```python
from build123d import *

# Parameters (mm, degrees)
SKETCH1_W           = 14.1
SKETCH1_H           = 31.1
BOSS_EXTRUDE1_DEPTH = 1.5
SKETCH2_W           = 10
SKETCH2_H           = 5.6
BOSS_EXTRUDE2_DEPTH = 9
SKETCH3_W           = 0.5
SKETCH3_H           = 5.6
BOSS_EXTRUDE3_DEPTH = 2.3
SKETCH4_R           = 1.5
BOSS_EXTRUDE4_DEPTH = 1.7
CHAMFER1_SIZE       = 1
CHAMFER2_SIZE       = 0.5
FILLET1_R           = 1
FILLET2_R           = 1
SKETCH5_R           = 0.4
BOSS_EXTRUDE5_DEPTH = 1
SKETCH6_R           = 1.5
CUT_EXTRUDE1_DEPTH  = 11


with BuildPart() as part:
    # Sketch1 → Boss-Extrude1 (new body)
    with BuildSketch(Plane(origin=(0, 0, 0), x_dir=(1, 0, 0), z_dir=(0, 1, 0))):
        Rectangle(SKETCH1_W, SKETCH1_H)
    extrude(amount=BOSS_EXTRUDE1_DEPTH)

    # Sketch2 → Boss-Extrude2 (add)
    with BuildSketch(Plane(origin=(0, 1.5, 0), x_dir=(1, 0, 0), z_dir=(0, 1, 0))):
        with Locations((0, 11.95)):
            Rectangle(SKETCH2_W, SKETCH2_H)
    extrude(amount=BOSS_EXTRUDE2_DEPTH)

    # Sketch3 → Boss-Extrude3 (add)
    with BuildSketch(Plane(origin=(0, 10.5, 0), x_dir=(1, 0, 0), z_dir=(0, 1, 0))):
        with Locations((0, 11.95)):
            Rectangle(SKETCH3_W, SKETCH3_H)
    extrude(amount=BOSS_EXTRUDE3_DEPTH)

    # Sketch4 → Boss-Extrude4 (add)
    with BuildSketch(Plane(origin=(0, 10.5, 0), x_dir=(1, 0, 0), z_dir=(0, 1, 0))):
        with Locations(Location((-2.625, 11.95, 0), (0, 0, 270))):
            Circle(SKETCH4_R)
        with Locations(Location((2.625, 11.95, 0), (0, 0, 270))):
            Circle(SKETCH4_R)
    extrude(amount=BOSS_EXTRUDE4_DEPTH)

    # Chamfer1
    chamfer1_edges = [part.edges().sort_by_distance(p)[0] for p in [
        (5, 6, -9.15),
        (5, 6, -14.75),
        (-5, 6, -14.75),
        (-5, 6, -9.15),
    ]]
    chamfer(chamfer1_edges, length=CHAMFER1_SIZE)

    # Chamfer2
    chamfer2_edges = [part.edges().sort_by_distance(p)[0] for p in [
        (-2.125, 10.5, -14.75),
        (2.125, 10.5, -9.15),
        (-5, 10.5, -11.95),
        (2.125, 10.5, -14.75),
        (-2.125, 10.5, -9.15),
        (-4.5, 10.5, -9.65),
        (-4.5, 10.5, -14.25),
        (5, 10.5, -11.95),
        (4.5, 10.5, -14.25),
        (4.5, 10.5, -9.65),
    ]]
    chamfer(chamfer2_edges, length=CHAMFER2_SIZE)

    # Fillet1
    fillet1_edges = [part.edges().sort_by_distance(p)[0] for p in [
        (-2.625, 12.2, -13.45),
        (2.625, 12.2, -13.45),
    ]]
    fillet(fillet1_edges, radius=FILLET1_R)

    # Fillet2
    fillet2_edges = [part.edges().sort_by_distance(p)[0] for p in [
        (0, 12.8, -14.75),
        (0, 12.8, -9.15),
    ]]
    fillet(fillet2_edges, radius=FILLET2_R)

    # Sketch5 → Boss-Extrude5 (add)
    with BuildSketch(Plane(origin=(0, 1.5, 0), x_dir=(1, 0, 0), z_dir=(0, 1, 0))):
        with Locations(Location((-4.05, 1.85, 0), (0, 0, 270))):
            Circle(SKETCH5_R)
        with Locations(Location((-1.55, -0.45, 0), (0, 0, 270))):
            Circle(SKETCH5_R)
        with Locations(Location((-4.05, -2.75, 0), (0, 0, 270))):
            Circle(SKETCH5_R)
        with Locations(Location((-3.84, -14.05, 0), (0, 0, 270))):
            Circle(SKETCH5_R)
        with Locations(Location((-1.28, -14.05, 0), (0, 0, 270))):
            Circle(SKETCH5_R)
        with Locations(Location((1.28, -14.05, 0), (0, 0, 270))):
            Circle(SKETCH5_R)
        with Locations(Location((3.84, -14.05, 0), (0, 0, 270))):
            Circle(SKETCH5_R)
    extrude(amount=BOSS_EXTRUDE5_DEPTH)

    # Sketch6 → Cut-Extrude1 (cut)
    with BuildSketch(Plane(origin=(0, 1.5, 0), x_dir=(1, 0, 0), z_dir=(0, 1, 0))):
        with Locations(Location((0, -8.55, 0), (0, 0, 270))):
            Circle(SKETCH6_R)
    extrude(amount=-CUT_EXTRUDE1_DEPTH, mode=Mode.SUBTRACT)


solid = part.part
```
Build history of the part. All positions in model axes, mm. A direction names the side the tool comes from. Round coordinates to 2 decimals unless told otherwise and drop trailing zeros. Write each loop counter-clockwise with the first axis right and the second up, starting at its lowest first coordinate (ties: lowest second). Pieces come first, ordered by that corner, then holes. Notation, with made-up numbers: (41, 66) -> (63, 66) arc R24 cw to (63, 91) -> close; hole circle Ø11 at (-31, 12). An arc over 180 degrees is marked (long way). Put each result on its own line as item: value.
Item 1: Slice it at C-C, the plane z = 11. Give the cut face in (x, y), plus the area to 4 significant figures.
Here are the results:
outline: (-7.05, 0) -> (7.05, 0) -> (7.05, 1.5) -> (-7.05, 1.5) -> close
area: 21.15 mm^2
Item 2: Two-plate mould, pull along X, no slides. Class faces 4 (the face through (-1, 10.5, -13)), 5 (the face through (7.05, 1, 0)), 6 (the face through (0.004, 12.499, -9.435)): pulls with the +X half, pulls with the -X half, needs draft (parallel to the pull), parting line crosses it, or undercut.
Here are the results:
face 4: undercut
face 5: pulls with the +X half
face 6: needs draft
Item 3: Wall check: probe 1 along X at (y, z) = (1.05, 8.55); probe 2 along Y at (x, z) = (-1.75, -1.5); probe 3 along Z at (x, y) = (-2.5, 2.5). Give the ranges that are in metal, low to high. Write a range as from..to.
Here are the results:
probe 1: x = -7.05..-1.5, 1.5..7.05
probe 2: y = 0..1.5
probe 3: z = -14.75..-9.15
Item 4: Slice it at B-B, the plane y = 5.25. Give the cut face in (x, z).
Here are the results:
outline: (-5, -13.75) -> (-4, -14.75) -> (4, -14.75) -> (5, -13.75) -> (5, -10.15) -> (4, -9.15) -> (-4, -9.15) -> (-5, -10.15) -> close
Item 5: Slice it at A-A, the plane z = 2.75. Give the cut face in (x, y).
Here are the results:
outline: (-7.05, 0) -> (7.05, 0) -> (7.05, 1.5) -> (-3.65, 1.5) -> (-3.65, 2.5) -> (-4.45, 2.5) -> (-4.45, 1.5) -> (-7.05, 1.5) -> close
Item 6: Tool access for faces 1 (the face through (-5, 6, -12)), 2 (the face through (3.86, 1.99, 13.65)), 3 (the face through (4.49, 5.69, -14.26)): list every direction of +Z, -Z, +X, -X, +Y, -Y with a clear straight run to the whole face (end or side of a thin tool).
Here are the results:
face 1: +Z, -Z, -X, +Y
face 2: +Y
face 3: -Z, +X, +Y
Item 7: Flat gauge pins, fed straight in: P1, Ø0.8, axis at y = 11.5, z = -13.5, coming from the -X side; P2, Ø3, axis at x = -0.5, y = 9, coming from the +Z side; P3, Ø1.8, axis at y = 4, z = -12, coming from the +X side; P4, Ø1, axis at y = 4, z = 4.5, coming from the +X side. Where does each tip first touch, or does it go through?
Here are the results:
P1: stops at x = -3.54
P2: stops at z = -9.15
P3: stops at x = 5
P4: passes through
